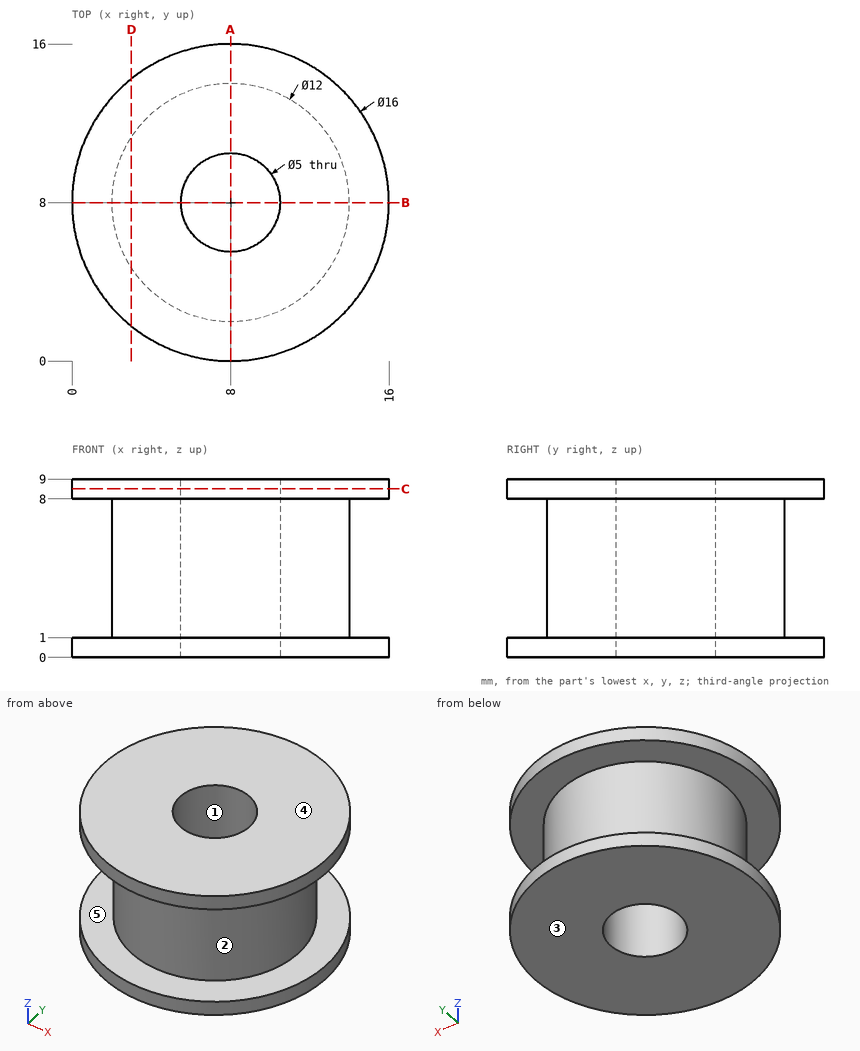
The drawing under review shows one solid part. Ordinate dimensions are in mm from its lowest x, y, z. A direction names the side the tool comes from. Round coordinates to 2 decimals unless told otherwise and drop trailing zeros. Loops run counter-clockwise (first coordinate to the right, second up) from the corner with the lowest first, then second, coordinate; pieces in that order, holes last. Notation, with made-up numbers: (40.5, -9.5) - (46.5, -9.5) arc R29 cw to (46.5, 25.5) - close; hole circle Ø9 at (-35, 66). An arc over 180 degrees is marked (long way). Use one line per item in the form item = value.
Item 1: Tool access review of the marked faces 4 and 5: name each direction out of +Z, -Z, +X, -X, +Y, -Y from which nothing blocks a thin tool from reaching the whole face with its end or side.
Answers:
face_4 = +Z, +X, -X, +Y, -Y
face_5 = none
Item 2: For line 1 (Y direction, x = 8, z = 6); line 2 (Z direction, x = 1.25, y = 7.75); line 3 (X direction, y = 5.75, z = 3.5), list the stretches that pass through material, from the lowest coordinate up.
Answers:
line_1 = 2 to 5.5, 10.5 to 14
line_2 = 0 to 1, 8 to 9
line_3 = 2.44 to 6.91, 9.09 to 13.56
Item 3: Clearance check with flat-ended pins moving along their axes: P1, Ø4, axis at x = 6, z = 6.5, coming from the +Y side; P2, Ø2, axis at x = 8.5, z = 2.5, coming from the +Y side. State where each tip first meets the part, or that it passes through.
Answers:
P1 = 15.97
P2 = 14
Item 4: Consider section D-D on x = 3. Write out the cut boundary in (y, z) (3 decimals), then the cut area to 3 significant figures.
Answers:
outline = (1.755, 0) - (14.245, 0) - (14.245, 1) - (11.317, 1) - (11.317, 8) - (14.245, 8) - (14.245, 9) - (1.755, 9) - (1.755, 8) - (4.683, 8) - (4.683, 1) - (1.755, 1) - close
area = 71.4 mm^2
Item 5: Mouldability with a two-part tool opening along Y and no side actions: class the marked faces 1, 2 and 3 as +Y half, -Y half, draft (parallel to the pull), parting line (faces both ways), or undercut.
Answers:
face_1 = undercut
face_2 = parting line
face_3 = draft
Item 6: Consider section C-C on z = 8.5. Write out the cut boundary in (x, y), then the cut area to 3 significant figures.
Answers:
outline = circle Ø16 at (8, 8); hole circle Ø5 at (8, 8)
area = 181 mm^2
Item 7: Consider section A-A on x = 8. Write out the cut boundary in (y, z).
Answers:
outline = (0, 0) - (5.5, 0) - (5.5, 9) - (0, 9) - (0, 8) - (2, 8) - (2, 1) - (0, 1) - close; (10.5, 0) - (16, 0) - (16, 1) - (14, 1) - (14, 8) - (16, 8) - (16, 9) - (10.5, 9) - close
